Verification items for the finished model (mm, model axes). A direction names the side the tool comes from. Round coordinates to 2 decimals unless told otherwise and drop trailing zeros. Write each loop counter-clockwise with the first axis right and the second up, starting at its lowest first coordinate (ties: lowest second). Pieces come first, ordered by that corner, then holes. Notation, with made-up numbers: (50, 87.25) - (80, 87.25) arc R13 ccw to (80, 107.25) - close; hole circle Ø9 at (-39.5, -35). An arc over 180 degrees is marked (long way). Answer as a JSON object with one key per item and string values. Group by question number.
1) Go/stop test with flat-tipped pins: pin 1 Ø24 at (x, z) = (3.5, -10) entering from +Y; pin 2 Ø12 at (x, z) = (-30, -30) entering from +Y; pin 3 Ø10 at (x, z) = (-4, 1.5) entering from -Y; pin 4 Ø23.5 at (x, z) = (25.5, -34.5) entering from -Y. Record where each tip stops, or that it passes through.
2) Thickness scan on line 1 (Z direction, x = -30, y = -14); line 2 (Z direction, x = 29, y = -14); line 3 (Y direction, x = -1, z = 12). Record the ranges inside material, lowest first.
3) Mould release check, pull along X, two halves, no side actions. Record for faces 1 (the conical face through (-0.308, -13.153, -18.362)), 2 (the cylindrical face through (3.3, -13.7, -21.1)), 3 (the cylindrical face through (-38.859, -12.675, 38.797)), 4 (the cylindrical face through (-19.524, -37.451, 4.336)): +X half, -X half, draft (parallel to the pull), parting line (faces both ways), or undercut.
4) Section check C-C (x = 30). Enter the section's corners in (y, z).
5) Section check B-B (z = -30). Enter the section's corners in (x, y).
6) Section check D-D (z = 30). Enter the section's corners in (x, y).
7) Set-up check for faces 5 (the cylindrical face through (-38.859, -12.675, -38.797)), 6 (the cylindrical face through (-11.107, 3.972, 26.789)), 7 (the cylindrical face through (23.69, -27.54, 24.03)), 8 (the flat face through (10.2, -2, -0.1)), 9 (the cylindrical face through (-9.76, -23.8, 2.17)): record each of +Z, -Z, +X, -X, +Y, -Y from which the full face is reachable in a straight line by a thin tool's end or side.
```python
from build123d import *

# Parameters (mm, degrees)
ESQUISSE1_R                  = 31.5
ESQUISSE1_R_2                = 29
BOSS_EXTRU_1_DEPTH           = 6
ESQUISSE2_R                  = 29
BOSS_EXTRU_2_DEPTH           = 2
ESQUISSE3_W                  = 80
ESQUISSE3_H                  = 80
BOSS_EXTRU_3_DEPTH           = 30
CONG_1_R                     = 4
ESQUISSE6_R                  = 20
BOSS_EXTRU_5_DEPTH           = 15
CONG_3_R                     = 4
ESQUISSE7_R                  = 10
ENL_V_MAT_EXTRU_2_DEPTH      = 77.164296097
ESQUISSE8_R                  = 17.170805795
ENL_V_MAT_EXTRU_3_DEPTH      = 5
ESQUISSE9_R                  = 3.731879986
ENL_V_MAT_EXTRU_4_DEPTH      = 65.505813816
R_P_TITION_CIRCULAIRE1_COUNT = 4
D_GAGEMENT_M61_D             = 6.6
D_GAGEMENT_M61_DEPTH         = 20
D_GAGEMENT_M61_TIP           = 1.982840043
D_GAGEMENT_M62_D             = 6.6
D_GAGEMENT_M62_DEPTH         = 20
D_GAGEMENT_M62_TIP           = 1.982840043
ESQUISSE14_R                 = 6
ENL_V_MAT_EXTRU_5_DEPTH      = 2
ESQUISSE15_R                 = 12.5
ENL_V_MAT_EXTRU_6_DEPTH      = 2


with BuildPart() as part:
    # Esquisse1 → Boss.-Extru.1 (new body)
    with BuildSketch(Plane(origin=(0, 0, 0), x_dir=(1, 0, 0), z_dir=(0, 1, 0))):
        with Locations(Location((0, 0, 0), (0, 0, 270))):
            Circle(ESQUISSE1_R)
        with Locations(Location((0, 0, 0), (0, 0, 270))):
            Circle(ESQUISSE1_R_2, mode=Mode.SUBTRACT)
    extrude(amount=BOSS_EXTRU_1_DEPTH)

    # Esquisse2 → Boss.-Extru.2 (add)
    with BuildSketch(Plane(origin=(0, 0, 0), x_dir=(1, 0, 0), z_dir=(0, 1, 0))):
        with Locations(Location((0, 0, 0), (0, 0, 270))):
            Circle(ESQUISSE2_R)
    extrude(amount=BOSS_EXTRU_2_DEPTH)

    # Esquisse3 → Boss.-Extru.3 (add)
    with BuildSketch(Plane.XZ):
        Rectangle(ESQUISSE3_W, ESQUISSE3_H)
    extrude(amount=BOSS_EXTRU_3_DEPTH)

    # Congé1
    cong_1_edges = [part.edges().sort_by_distance(p)[0] for p in [
        (-40, -15, 40),
        (-40, -15, -40),
        (40, -15, -40),
        (40, -15, 40),
        (-40, -30, 0),
        (0, -30, -40),
        (40, -30, 0),
        (0, -30, 40),
    ]]
    fillet(cong_1_edges, radius=CONG_1_R)

    # Esquisse6 → Boss.-Extru.5 (add)
    with BuildSketch(Plane.XZ.offset(30)):
        with Locations(Location((0, 0, 0), (0, 0, 270))):
            Circle(ESQUISSE6_R)
    extrude(amount=BOSS_EXTRU_5_DEPTH)

    # Congé3
    cong_3_edges = [part.edges().sort_by_distance(p)[0] for p in [
        (0, -30, 20),
        (0, -45, 20),
    ]]
    fillet(cong_3_edges, radius=CONG_3_R)

    # Esquisse7 → Enlèv. mat.-Extru.2 (cut, through all)
    with BuildSketch(Plane(origin=(0, -45, 0), x_dir=(-1, 0, 0), z_dir=(0, -1, 0))):
        with Locations(Location((0, 0, 0), (0, 0, 90))):
            Circle(ESQUISSE7_R)
    extrude(amount=-ENL_V_MAT_EXTRU_2_DEPTH, mode=Mode.SUBTRACT)

    # Esquisse8 → Enlèv. mat.-Extru.3 (cut)
    with BuildSketch(Plane.XZ.offset(30)):
        with Locations((36, -36)):
            Circle(ESQUISSE8_R)
    enl_v_mat_extru_3 = extrude(amount=-ENL_V_MAT_EXTRU_3_DEPTH, mode=Mode.SUBTRACT)

    # Esquisse9 → Enlèv. mat.-Extru.4 (cut, through all)
    with BuildSketch(Plane.XZ.offset(25)):
        with Locations(Location((30, -30, 0), (0, 0, 270))):
            Circle(ESQUISSE9_R)
    enl_v_mat_extru_4 = extrude(amount=-ENL_V_MAT_EXTRU_4_DEPTH, mode=Mode.SUBTRACT)

    # Répétition circulaire1: Enlèv. mat.-Extru.3, Enlèv. mat.-Extru.4 ×4 about axis
    r_p_tition_circulaire1_axis = Axis((0, 0, 0), (0, 1, 0))
    add([enl_v_mat_extru_3.rotate(r_p_tition_circulaire1_axis, i * 360 / R_P_TITION_CIRCULAIRE1_COUNT) for i in range(1, R_P_TITION_CIRCULAIRE1_COUNT)], mode=Mode.SUBTRACT)
    add([enl_v_mat_extru_4.rotate(r_p_tition_circulaire1_axis, i * 360 / R_P_TITION_CIRCULAIRE1_COUNT) for i in range(1, R_P_TITION_CIRCULAIRE1_COUNT)], mode=Mode.SUBTRACT)

    # Dégagement M61
    with Locations(Plane(origin=(0, 2, 0), x_dir=(1, 0, 0), z_dir=(0, 1, 0))):
        with Locations((0, 22.784568399)):
            Hole(D_GAGEMENT_M61_D / 2, depth=D_GAGEMENT_M61_DEPTH)
            with Locations((0, 0, -(D_GAGEMENT_M61_DEPTH + D_GAGEMENT_M61_TIP / 2))):  # 118° drill point
                Cone(0, D_GAGEMENT_M61_D / 2, D_GAGEMENT_M61_TIP, mode=Mode.SUBTRACT)

    # Dégagement M62
    with Locations(Plane(origin=(0, 0, -40), x_dir=(-1, 0, 0), z_dir=(0, 0, -1))):
        with Locations((0, -13.635863914)):
            Hole(D_GAGEMENT_M62_D / 2, depth=D_GAGEMENT_M62_DEPTH)
            with Locations((0, 0, -(D_GAGEMENT_M62_DEPTH + D_GAGEMENT_M62_TIP / 2))):  # 118° drill point
                Cone(0, D_GAGEMENT_M62_D / 2, D_GAGEMENT_M62_TIP, mode=Mode.SUBTRACT)

    # Esquisse14 → Enlèv. mat.-Extru.5 (cut)
    with BuildSketch(Plane(origin=(0, 0, -40), x_dir=(-1, 0, 0), z_dir=(0, 0, -1))):
        with Locations((0, -13.635863914)):
            Circle(ESQUISSE14_R)
    extrude(amount=-ENL_V_MAT_EXTRU_5_DEPTH, mode=Mode.SUBTRACT)

    # Esquisse15 → Enlèv. mat.-Extru.6 (cut)
    with BuildSketch(Plane(origin=(0, 0, 0), x_dir=(1, 0, 0), z_dir=(0, 1, 0))):
        with Locations(Location((0, 0, 0), (0, 0, 270))):
            Circle(ESQUISSE15_R)
    extrude(amount=-ENL_V_MAT_EXTRU_6_DEPTH, mode=Mode.SUBTRACT)


solid = part.part
```
Returned:
{
 "1": {"pin 1": "y = 2", "pin 2": "y = 0", "pin 3": "through", "pin 4": "y = -30"},
 "2": {"line 1": "-40 to -33.73, -26.27 to 26.27, 33.73 to 40", "line 2": "-40 to -33.6, -26.4 to 26.4, 33.6 to 40", "line 3": "-45 to -2, 0 to 2"},
 "3": {"face 1": "undercut", "face 2": "undercut", "face 3": "-X half", "face 4": "parting line"},
 "4": {"outline": "(-30, -19.91) - (-25, -19.91) - (-25, -26.27) - (0, -26.27) - (0, -9.6) - (6, -9.6) - (6, 9.6) - (0, 9.6) - (0, 26.27) - (-25, 26.27) - (-25, 19.91) - (-30, 19.91) - close; (-25, -40) - (0, -40) - (0, -33.73) - (-25, -33.73) - close; (-25, 33.73) - (0, 33.73) - (0, 40) - (-25, 40) - close"},
 "5": {"outline": "(-40, -25) - (-33.73, -25) - (-33.73, 0) - (-40, 0) - close; (-26.27, -25) - (-19.91, -25) - (-19.91, -30) - (19.91, -30) - (19.91, -25) - (26.27, -25) - (26.27, 0) - (9.6, 0) - (9.6, 6) - (-9.6, 6) - (-9.6, 0) - (-26.27, 0) - close; (33.73, -25) - (40, -25) - (40, 0) - (33.73, 0) - close; hole circle Ø6.6 at (0, -13.64)"},
 "6": {"outline": "(-40, -25) - (-33.73, -25) - (-33.73, 0) - (-40, 0) - close; (-26.27, -25) - (-19.91, -25) - (-19.91, -30) - (19.91, -30) - (19.91, -25) - (26.27, -25) - (26.27, 0) - (9.6, 0) - (9.6, 6) - (-9.6, 6) - (-9.6, 0) - (-26.27, 0) - close; (33.73, -25) - (40, -25) - (40, 0) - (33.73, 0) - close"},
 "7": {"face 5": "-Z, -X, +Y, -Y", "face 6": "+Y", "face 7": "-Y", "face 8": "none", "face 9": "+Y, -Y"}
}
